CAD build for the part. Positions are in the model's coordinates, mm. Face numbers are marked on the shaded views. Give positions to 0.01 mm unless a question says otherwise; leave off trailing zeros. Write each loop counter-clockwise with the first axis right and the second up, starting at its lowest first coordinate (ties: lowest second). Pieces come first, ordered by that corner, then holes. Notation, with made-up numbers: (48, 61.5) - (83, 61.5) arc R23 ccw to (83, 96.5) - close; hole circle Ø11 at (7.25, -16). An arc over 180 degrees is marked (long way). Answer as a JSON object with one key per item and string values.
from build123d import *

# Parameters (mm, degrees)
ENL_V_MAT_EXTRU_1_DEPTH = 2
CHANFREIN1_SIZE         = 0.2


with BuildPart() as part:
    # Esquisse1 → Révolution1 (revolve)
    with BuildSketch(Plane.XY):
        Polygon((0, 0), (0, 3), (0.2, 3), (1.7, 1.5), (7.7, 1.5), (7.7, 0), align=None)
    revolve(axis=Axis((0, 0, 0), (1, 0, 0)))

    # Esquisse2 → Enlèv. mat.-Extru.1 (cut)
    with BuildSketch(Plane.ZY):
        Polygon((0.433012702, -0.75), (0.866025404, 0), (0.433012702, 0.75), (-0.433012702, 0.75), (-0.866025404, 0), (-0.433012702, -0.75), align=None)
    extrude(amount=-ENL_V_MAT_EXTRU_1_DEPTH, mode=Mode.SUBTRACT)

    # Chanfrein1
    chanfrein1_edges = [part.edges().sort_by_distance(p)[0] for p in [
        (7.7, -1.5, 0),
    ]]
    chamfer(chanfrein1_edges, length=CHANFREIN1_SIZE)


solid = part.part
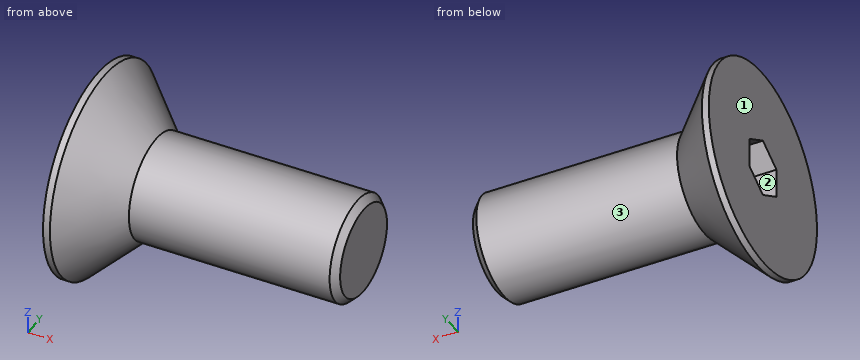
(1) Flat gauge pins, fed straight in: P1, Ø1, axis at x = 1, z = 0, coming from the -Y side; P2, Ø1, axis at x = 1.5, z = 0, coming from the +Y side; P3, Ø1.5, axis at x = 7, y = -1.5, coming from the -Z side. Where does each tip first touch, or does it go through?
Answer key:
{"P1": "stops at y = -2.7", "P2": "stops at y = 2.2", "P3": "stops at z = -1.3"}
(2) Saw through at A-A, the plane z = 0. Give the cut face in (x, y), and give its area (3 significant figures).
Answer key:
{"outline": "(0, -3) - (0.2, -3) - (1.7, -1.5) - (7.5, -1.5) - (7.7, -1.3) - (7.7, 1.3) - (7.5, 1.5) - (1.7, 1.5) - (0.2, 3) - (0, 3) - (0, 0.75) - (2, 0.75) - (2, -0.75) - (0, -0.75) - close", "area": "22.9 mm²"}
(3) Pull direction Y, two halves, no side cores. Call the marked faces 1, 2 and 3: pulls with the +Y half, pulls with the -Y half, needs draft (parallel to the pull), parting line crosses it, or undercut.
Answer key:
{"face 1": "needs draft", "face 2": "undercut", "face 3": "parting line crosses it"}
(4) Saw through at B-B, the plane x = 2.25. Give the cut face in (y, z), and give its area (3 significant figures).
Answer key:
{"outline": "circle Ø3 at (0, 0)", "area": "7.07 mm²"}
(5) Probe L1, parallel to Z at x = 2.5, y = 0; L2, parallel to X at y = 0.1, z = -0.55; L3, parallel to Z at x = 1.25, y = -0.5. List the from-to ranges inside material, lowest first. Write a range as [from, to].
Answer key:
{"L1": "z = [-1.5, 1.5]", "L2": "x = [2, 7.7]", "L3": "z = [-1.88, -0.58], [0.58, 1.88]"}
